from build123d import *

# Parameters (mm, degrees)
SKETCH1_W           = 40
SKETCH1_H           = 40
BOSS_EXTRUDE1_DEPTH = 2
SKETCH2_W           = 30
SKETCH2_H           = 30
SKETCH2_W_2         = 26
SKETCH2_H_2         = 26
BOSS_EXTRUDE2_DEPTH = 3
FILLET1_R           = 0.5
FILLET2_R           = 0.5
FILLET3_R           = 0.5


with BuildPart() as part:
    # Sketch1 → Boss-Extrude1 (new body)
    with BuildSketch(Plane.XY):
        with Locations((-5.192307692, 0.701169798)):
            Rectangle(SKETCH1_W, SKETCH1_H)
    extrude(amount=BOSS_EXTRUDE1_DEPTH)

    # Sketch2 → Boss-Extrude2 (add)
    with BuildSketch(Plane.XY.offset(2)):
        with Locations((-5.192307692, 0.701169798)):
            Rectangle(SKETCH2_W, SKETCH2_H)
        with Locations((-5.192307692, 0.701169798)):
            Rectangle(SKETCH2_W_2, SKETCH2_H_2, mode=Mode.SUBTRACT)
    extrude(amount=BOSS_EXTRUDE2_DEPTH)

    # Fillet1
    fillet1_edges = [part.edges().sort_by_distance(p)[0] for p in [
        (-20.192307692, 0.701169798, 5),
        (-5.192307692, -14.298830202, 5),
        (9.807692308, 0.701169798, 5),
        (-5.192307692, 15.701169798, 5),
        (-18.192307692, 0.701169798, 5),
        (-5.192307692, -12.298830202, 5),
        (7.807692308, 0.701169798, 5),
        (-5.192307692, 13.701169798, 5),
    ]]
    fillet(fillet1_edges, radius=FILLET1_R)

    # Fillet2
    fillet2_edges = [part.edges().sort_by_distance(p)[0] for p in [
        (14.807692308, 0.701169798, 2),
        (-5.192307692, 20.701169798, 2),
        (-25.192307692, 0.701169798, 2),
        (-5.192307692, 20.701169798, 0),
        (14.807692308, 0.701169798, 0),
        (-5.192307692, -19.298830202, 0),
        (-25.192307692, 0.701169798, 0),
        (-25.192307692, 20.701169798, 1),
        (14.807692308, 20.701169798, 1),
        (14.807692308, -19.298830202, 1),
        (-25.192307692, -19.298830202, 1),
        (-5.192307692, -19.298830202, 2),
    ]]
    fillet(fillet2_edges, radius=FILLET2_R)

    # Fillet3
    fillet3_edges = [part.edges().sort_by_distance(p)[0] for p in [
        (-20.192307692, 0.701169798, 2),
        (-5.192307692, -14.298830202, 2),
        (9.807692308, 0.701169798, 2),
        (-5.192307692, 15.701169798, 2),
    ]]
    fillet(fillet3_edges, radius=FILLET3_R)


solid = part.part
Input: part model. Units: mm. Frame: model coordinates. A direction names the side the tool comes from. Give positions to 0.01 mm unless a question says otherwise; leave off trailing zeros. Order: outer loops, then holes, each group sorted by start corner. A loop starts at its lowest first (then second) coordinate and runs counter-clockwise, first axis right, second up. Notation, with made-up numbers: (-40, 44) -> (-2, 44) arc R25 cw to (-2, 74) -> close; hole circle Ø4 at (75, 73). An arc over 180 degrees is marked (long way). Use one line per item in the form item = value.
1) Section A-A, the plane x = -21.5. Return loops of the section in (y, z).
Response values:
outline = (-19.3, 0.5) arc R0.5 ccw to (-18.8, 0) -> (20.2, 0) arc R0.5 ccw to (20.7, 0.5) -> (20.7, 1.5) arc R0.5 ccw to (20.2, 2) -> (-18.8, 2) arc R0.5 ccw to (-19.3, 1.5) -> close
2) Reachability of faces 5 (the flat face through (9.808, 0, 3)), 6 (the flat face through (-5, -14.299, 3)), 7 (the flat face through (-5, -12.299, 3)), 8 (the flat face through (-20.192, 0, 3)) from +Z, -Z, +X, -X, +Y, -Y: full face, straight path, thin tool, end or side. Return the list, or none.
Response values:
face_5 = +Z, +X, +Y, -Y
face_6 = +Z, +X, -X, -Y
face_7 = +Z
face_8 = +Z, -X, +Y, -Y
3) Section B-B, the plane z = 3.55. Return loops of the section in (x, y), and give its area (3 significant figures).
Response values:
outline = (-20.19, -14.3) -> (9.81, -14.3) -> (9.81, 15.7) -> (-20.19, 15.7) -> close; hole (-18.19, -12.3) -> (7.81, -12.3) -> (7.81, 13.7) -> (-18.19, 13.7) -> close
area = 224 mm^2
4) Line query: probe 1 along Y at (x, z) = (-10, 3.45); probe 2 along X at (y, z) = (-3.5, 4.4); probe 3 along Z at (x, y) = (-18, 11). Output: solid intervals per line, ascending.
Response values:
probe_1 = -14.3 to -12.3, 13.7 to 15.7
probe_2 = -20.19 to -18.19, 7.81 to 9.81
probe_3 = 0 to 2
5) First-contact query: pin 1 Ø1.6 at (y, z) = (3, 4) entering from +X; pin 2 Ø3 at (y, z) = (-5, 4) entering from -X; pin 3 Ø0.8 at (x, z) = (-6.5, 3) entering from +Y. Flat tips, straight axial feed; report the tip coordinate or a pass-through.
Response values:
pin_1 = 9.81
pin_2 = -20.19
pin_3 = 15.7
6) Section C-C, the plane y = -6. Return loops of the section in (x, z).
Response values:
outline = (-25.19, 0.5) arc R0.5 ccw to (-24.69, 0) -> (14.31, 0) arc R0.5 ccw to (14.81, 0.5) -> (14.81, 1.5) arc R0.5 ccw to (14.31, 2) -> (10.31, 2) arc R0.5 cw to (9.81, 2.5) -> (9.81, 4.5) arc R0.5 ccw to (9.31, 5) -> (8.31, 5) arc R0.5 ccw to (7.81, 4.5) -> (7.81, 2) -> (-18.19, 2) -> (-18.19, 4.5) arc R0.5 ccw to (-18.69, 5) -> (-19.69, 5) arc R0.5 ccw to (-20.19, 4.5) -> (-20.19, 2.5) arc R0.5 cw to (-20.69, 2) -> (-24.69, 2) arc R0.5 ccw to (-25.19, 1.5) -> close
7) Mould query, pull axis Y, two halves, no side actions, for faces 1 (the flat face through (-5, -19.299, 1)), 2 (the flat face through (12, 1, 2)), 3 (the flat face through (-18.192, 1, 3)), 4 (the flat face through (-5, 15.701, 3)). Classes: pulls with the +Y half, pulls with the -Y half, needs draft (parallel to the pull), parting line crosses it, or undercut.
Response values:
face_1 = pulls with the -Y half
face_2 = needs draft
face_3 = undercut
face_4 = pulls with the +Y half
8) Section D-D, the plane x = 6. Return loops of the section in (y, z), and give its area (3 significant figures).
Response values:
outline = (-19.3, 0.5) arc R0.5 ccw to (-18.8, 0) -> (20.2, 0) arc R0.5 ccw to (20.7, 0.5) -> (20.7, 1.5) arc R0.5 ccw to (20.2, 2) -> (16.2, 2) arc R0.5 cw to (15.7, 2.5) -> (15.7, 4.5) arc R0.5 ccw to (15.2, 5) -> (14.2, 5) arc R0.5 ccw to (13.7, 4.5) -> (13.7, 2) -> (-12.3, 2) -> (-12.3, 4.5) arc R0.5 ccw to (-12.8, 5) -> (-13.8, 5) arc R0.5 ccw to (-14.3, 4.5) -> (-14.3, 2.5) arc R0.5 cw to (-14.8, 2) -> (-18.8, 2) arc R0.5 ccw to (-19.3, 1.5) -> close
area = 91.7 mm^2
